from build123d import *

# Parameters (mm, degrees)
CUT_EXTRUDE1_DEPTH = 5.08
CIRPATTERN1_COUNT  = 3


# Read off the part's stored shape, not the designer's step: Revolve1
with BuildPart() as part:
    # Revolve1 outline → Revolve1 (revolve)
    with BuildSketch(Plane.YX):
        Polygon((20.701, 0), (20.701, 7.62), (16.51, 7.62), (16.51, 88.9), (15.875, 88.9), (15.875, 76.2), (15.24, 76.2), (15.24, 5.08), (18.161, 5.08), (18.161, 0), align=None)
    revolve(axis=Axis((0, 0, 0), (1, 0, 0)))

    # Sketch2 → Cut-Extrude1 (cut)
    with BuildSketch(Plane(origin=(0, 16.51, 0), x_dir=(1, 0, 0), z_dir=(0, 1, 0))):
        with BuildLine():
            Line((20.6375, 3.175), (20.6375, -3.175))
            ThreePointArc((20.6375, -3.175), (19.05, -4.7625), (17.4625, -3.175))
            Line((17.4625, -3.175), (17.4625, 3.175))
            ThreePointArc((17.4625, 3.175), (19.05, 4.7625), (20.6375, 3.175))
        make_face()
    cut_extrude1 = extrude(amount=-CUT_EXTRUDE1_DEPTH, mode=Mode.SUBTRACT)

    # CirPattern1: Cut-Extrude1 ×3 about axis
    cirpattern1_axis = Axis((0, 0, 0), (1, 0, 0))
    for i in range(1, CIRPATTERN1_COUNT):
        add(cut_extrude1.rotate(cirpattern1_axis, i * 360 / CIRPATTERN1_COUNT), mode=Mode.SUBTRACT)


solid = part.part
Could you check a few things on this model? Use its own coordinates, in mm. A direction names the side the tool comes from. Give positions to 0.01 mm unless a question says otherwise; leave off trailing zeros. Loops run counter-clockwise (first coordinate to the right, second up) from the corner with the lowest first, then second, coordinate; pieces in that order, holes last. Notation, with made-up numbers: (5, 48.25) -> (39, 48.25) arc R17 ccw to (39, 60.25) -> close; hole circle Ø5 at (-17, 10). An arc over 180 degrees is marked (long way). Return JSON: item names as keys, results as strings.
Item 1: If we section it at B-B on x = 19.05: List the corners of the cut face in (y, z) for me.
Geometry results:
{"outline": "(-12.03, -11.31) -> (-11.36, -10.16) arc R15.24 cw to (-11.36, 10.16) -> (-12.03, 11.31) arc R16.51 ccw to start; (-3.78, -16.07) arc R16.51 ccw to (15.81, -4.76) -> (14.48, -4.76) arc R15.24 cw to (-3.11, -14.92) -> close; (-3.78, 16.07) -> (-3.11, 14.92) arc R15.24 cw to (14.48, 4.76) -> (15.81, 4.76) arc R16.51 ccw to start"}
Item 2: If we section it at C-C on y = 0: List the corners of the cut face in (x, z) for me (3 decimals).
Geometry results:
{"outline": "(0, -20.701) -> (7.62, -20.701) -> (7.62, -16.51) -> (88.9, -16.51) -> (88.9, -15.875) -> (76.2, -15.875) -> (76.2, -15.24) -> (5.08, -15.24) -> (5.08, -18.161) -> (0, -18.161) -> close; (0, 18.161) -> (5.08, 18.161) -> (5.08, 15.24) -> (76.2, 15.24) -> (76.2, 15.875) -> (88.9, 15.875) -> (88.9, 16.51) -> (7.62, 16.51) -> (7.62, 20.701) -> (0, 20.701) -> close"}
Item 3: Which directions (+Z, -Z, +X, -X, +Y, -Y) give clear straight access to the entire face, cutting with the end or side of a thin tool? Please do faces 4 (the flat face through (20.638, 16, 0)), 5 (the cylindrical face through (19.08, -11.8, 10.91)), 6 (the cylindrical face through (19.02, -11.8, -10.91)).
Geometry results:
{"face 4": "+Y", "face 5": "+Z", "face 6": "-Z"}
Item 4: We'd pull the mould along Y, two halves only. Please class faces 1 (the cylindrical face through (19.015, -3.552, 15.676)), 2 (the cylindrical face through (82.461, -3.441, -15.497)), 3 (the flat face through (7.62, -2, -17)): +Y half, -Y half, draft (parallel to the pull), parting line (faces both ways), or undercut.
Geometry results:
{"face 1": "-Y half", "face 2": "undercut", "face 3": "draft"}
Item 5: If we section it at D-D on x = 79: List the corners of the cut face in (y, z) for me (3 decimals), plus the area to 3 significant figures.
Geometry results:
{"outline": "circle Ø33.02 at (0, 0); hole circle Ø31.75 at (0, 0)", "area": "64.6 mm²"}
Item 6: I'm going to push flat-ended pins straight in: pin 1 (0.8 mm diameter, centred on y = 16, z = -1.5, fed in from -X); pin 2 (1.5 mm diameter, centred on x = 64.5, z = 6.5, fed in from +Y); pin 3 (8 mm diameter, centred on x = 50, y = -5.5, fed in from +Z). Where does each tip first touch, or does it pass through?
Geometry results:
{"pin 1": "stops at x = 5.08", "pin 2": "stops at y = 15.48", "pin 3": "stops at z = 16.44"}
Item 7: If we section it at A-A on z = 0: List the corners of the cut face in (x, y) for me (1 decimal), plus the area to 3 significant figures.
Geometry results:
{"outline": "(0, -20.7) -> (7.6, -20.7) -> (7.6, -16.5) -> (88.9, -16.5) -> (88.9, -15.9) -> (76.2, -15.9) -> (76.2, -15.2) -> (5.1, -15.2) -> (5.1, -18.2) -> (0, -18.2) -> close; (0, 18.2) -> (5.1, 18.2) -> (5.1, 15.2) -> (17.5, 15.2) -> (17.5, 16.5) -> (7.6, 16.5) -> (7.6, 20.7) -> (0, 20.7) -> close; (20.6, 15.2) -> (76.2, 15.2) -> (76.2, 15.9) -> (88.9, 15.9) -> (88.9, 16.5) -> (20.6, 16.5) -> close", "area": "240 mm²"}
Item 8: I need wall thicknesses on L1, parallel to Z at x = 73, y = 0.5; L2, parallel to X at y = -1.5, z = -16; L3, parallel to X at y = -16, z = 11. Which ranges of each line are inside material? Lowest first, please. Write a range as from..to.
Geometry results:
{"L1": "z = -16.5..-15.23, 15.23..16.5", "L2": "x = 5.08..88.9", "L3": "x = 0..7.62"}
